```python
from build123d import *

# Parameters (mm, degrees)
F0_W     = 43
F0_H     = 21
F0_R     = 1.65
F1_DEPTH = 1.6
F2_W     = 43
F2_H     = 11
F3_DEPTH = 11


with BuildPart() as f1:
    # F0 (on Top) → F1 (new body)
    with BuildSketch(Plane.XY):
        Rectangle(F0_W, F0_H)
        with Locations((15.5, -8)):
            Circle(F0_R, mode=Mode.SUBTRACT)
        with Locations((-15.5, 8)):
            Circle(F0_R, mode=Mode.SUBTRACT)
    extrude(amount=F1_DEPTH)

    # F2 (on face) → F3 (join)
    with BuildSketch(Plane.XY.offset(1.6)):
        Rectangle(F2_W, F2_H)
    extrude(amount=F3_DEPTH)


solid = f1.part
```
Work out the finished part from the listing and answer in its coordinate system (mm). A direction names the side the tool comes from. Coordinates: 2 decimals unless noted, no trailing zeros. Write each loop counter-clockwise with the first axis right and the second up, starting at its lowest first coordinate (ties: lowest second). Pieces come first, ordered by that corner, then holes.
Q1. Each of these flat-tipped pins is pushed along its axis until it touches: pin 1 Ø1 at (x, z) = (-13.5, 5) entering from -Y; pin 2 Ø4 at (x, y) = (7.5, -8.5) entering from +Z; pin 3 Ø5 at (x, z) = (-14.5, 8) entering from +Y. Where does it stop, or does it pass through?
Q2. Find the intervals of material crossed by line 1 (Y direction, x = 15.5, z = 1.1); line 2 (Y direction, x = -15.5, z = 0.8); line 3 (Z direction, x = 9, y = -8.75), in increasing order.
Q3. Determine the mould class of faces 4 (the face through (17.074, -7.504, 0.789)), 5 (the face through (0, -10.5, 1)), 6 (the face through (0, 5.5, 7)) for opening direction Y: released by +Y, released by -Y, zero draft, split by the parting line, or undercut.
Q4. A cutting plane is placed at B-B, the plane x = 15.5. Give the vertices of the cut face in (y, z).
Q5. A cutting plane is placed at A-A, the plane y = -8. Give the vertices of the cut face in (x, z), then the cut area to 3 significant figures.
Q6. Which of the six approach directions +Z, -Z, +X, -X, +Y, -Y give full straight-line access (tool end or side, diameter ignored) to faces 1 (the face through (-13.926, 8.496, 0.789)), 2 (the face through (0, -5.5, 7)), 3 (the face through (0, 8, 1.6))?
Q7. A cutting plane is placed at C-C, the plane z = 10.75. Give the vertices of the cut face in (x, y), then the cut area to 3 significant figures.
Findings below:
1. pin 1: stops at y = -5.5
1. pin 2: stops at z = 1.6
1. pin 3: stops at y = 5.5
2. line 1: y = -10.5 to -9.65, -6.35 to 10.5
2. line 2: y = -10.5 to 6.35, 9.65 to 10.5
2. line 3: z = 0 to 1.6
3. face 4: undercut
3. face 5: released by -Y
3. face 6: released by +Y
4. outline: (-10.5, 0) - (-9.65, 0) - (-9.65, 1.6) - (-10.5, 1.6) - close; (-6.35, 0) - (10.5, 0) - (10.5, 1.6) - (5.5, 1.6) - (5.5, 12.6) - (-5.5, 12.6) - (-5.5, 1.6) - (-6.35, 1.6) - close
5. outline: (-21.5, 0) - (13.85, 0) - (13.85, 1.6) - (-21.5, 1.6) - close; (17.15, 0) - (21.5, 0) - (21.5, 1.6) - (17.15, 1.6) - close
5. area: 63.5 mm2
6. face 1: +Z, -Z
6. face 2: +Z, +X, -X, -Y
6. face 3: +Z, +X, -X, +Y
7. outline: (-21.5, -5.5) - (21.5, -5.5) - (21.5, 5.5) - (-21.5, 5.5) - close
7. area: 473 mm2
